from build123d import *

# Parameters (mm, degrees)
SKETCH_1_W          = 72
SKETCH_1_H          = 16
EXTRUDE_1_DEPTH     = 1.2
FILLET_1_R          = 3
CUT_EXTRUDE_1_REACH = 75.766
SKETCH_3_R          = 1.2


with BuildPart() as part:
    # 草图1 → 凸台-拉伸1 (new body)
    with BuildSketch(Plane.XY):
        with Locations((36, 8)):
            Rectangle(SKETCH_1_W, SKETCH_1_H)
    extrude(amount=EXTRUDE_1_DEPTH)

    # 圆角1
    fillet_1_edges = [part.edges().sort_by_distance(p)[0] for p in [
        (0, 16, 0.6),
        (72, 16, 0.6),
        (72, 0, 0.6),
        (0, 0, 0.6),
    ]]
    fillet(fillet_1_edges, radius=FILLET_1_R)

    # 草图3 → 切除-拉伸1 (cut, up to next)
    with BuildSketch(Plane(origin=(0, 0, 0), x_dir=(-1, 0, 0), z_dir=(0, 0, -1)), mode=Mode.PRIVATE) as cut_extrude_1_sk1:
        with Locations((-70.012877826, 14.013032766)):
            Circle(SKETCH_3_R)
    cut_extrude_1_tool1 = extrude(cut_extrude_1_sk1.sketch, amount=-CUT_EXTRUDE_1_REACH, mode=Mode.PRIVATE) & part.part
    # 草图3 → 切除-拉伸1 (cut, up to next)
    with BuildSketch(Plane(origin=(0, 0, 0), x_dir=(-1, 0, 0), z_dir=(0, 0, -1)), mode=Mode.PRIVATE) as cut_extrude_1_sk2:
        with Locations((-70.012694945, 2.012672085)):
            Circle(SKETCH_3_R)
    cut_extrude_1_tool2 = extrude(cut_extrude_1_sk2.sketch, amount=-CUT_EXTRUDE_1_REACH, mode=Mode.PRIVATE) & part.part
    # 草图3 → 切除-拉伸1 (cut, up to next)
    with BuildSketch(Plane(origin=(0, 0, 0), x_dir=(-1, 0, 0), z_dir=(0, 0, -1)), mode=Mode.PRIVATE) as cut_extrude_1_sk3:
        with Locations((-2.011949988, 14.012003328)):
            Circle(SKETCH_3_R)
    cut_extrude_1_tool3 = extrude(cut_extrude_1_sk3.sketch, amount=-CUT_EXTRUDE_1_REACH, mode=Mode.PRIVATE) & part.part
    # 草图3 → 切除-拉伸1 (cut, up to next)
    with BuildSketch(Plane(origin=(0, 0, 0), x_dir=(-1, 0, 0), z_dir=(0, 0, -1)), mode=Mode.PRIVATE) as cut_extrude_1_sk4:
        with Locations((-2.012501905, 2.013009906)):
            Circle(SKETCH_3_R)
    cut_extrude_1_tool4 = extrude(cut_extrude_1_sk4.sketch, amount=-CUT_EXTRUDE_1_REACH, mode=Mode.PRIVATE) & part.part
    add(cut_extrude_1_tool1.solids().sort_by_distance((70.012878, 14.013033, 0))[0], mode=Mode.SUBTRACT)
    add(cut_extrude_1_tool2.solids().sort_by_distance((70.012695, 2.012672, 0))[0], mode=Mode.SUBTRACT)
    add(cut_extrude_1_tool3.solids().sort_by_distance((2.01195, 14.012003, 0))[0], mode=Mode.SUBTRACT)
    add(cut_extrude_1_tool4.solids().sort_by_distance((2.012502, 2.01301, 0))[0], mode=Mode.SUBTRACT)


solid = part.part
Part model, mm, in its own coordinate system. Give positions to 0.01 mm unless a question says otherwise; leave off trailing zeros. Order: outer loops, then holes, each group sorted by start corner. A loop starts at its lowest first (then second) coordinate and runs counter-clockwise, first axis right, second up. Notation, with made-up numbers: (25.5, 11) - (84.5, 11) arc R10 cw to (84.5, 22) - close; hole circle Ø10 at (42.5, 55.25). An arc over 180 degrees is marked (long way). Use a Markdown table: item, result.
1) Flat gauge pin, fed straight in: P1, Ø1.9, axis at x = 2.01, y = 14.01, coming from the -Z side. Where does the tip first touch, or does it go through?
Checked values:
| item | result |
|---|---|
| P1 | through |
2) Saw through at A-A on z = 0.5. List the corners of the cut face in (x, y), plus the area to 3 significant figures.
Checked values:
| item | result |
|---|---|
| outline | (0, 3) arc R3 ccw to (3, 0) - (69, 0) arc R3 ccw to (72, 3) - (72, 13) arc R3 ccw to (69, 16) - (3, 16) arc R3 ccw to (0, 13) - close; hole circle Ø2.4 at (2.01, 2.01); hole circle Ø2.4 at (2.01, 14.01); hole circle Ø2.4 at (70.01, 2.01); hole circle Ø2.4 at (70.01, 14.01) |
| area | 1,130 mm² |
3) Probe L1, parallel to X at y = 3, z = 0.1; L2, parallel to X at y = 15, z = 0.1. List the from-to ranges inside material, lowest first. Write a range as from..to.
Checked values:
| item | result |
|---|---|
| L1 | 0..1.33, 2.7..69.33, 70.69..72 |
| L2 | 0.76..1.33, 2.69..69.33, 70.7..71.24 |
4) Two-plate mould, pull along X, no slides. Class faces 1 (the flat face through (36, 0, 1)), 2 (the cylindrical face through (2.17, 15.2, 0.59)), 3 (the flat face through (0, 8, 1)): +X half, -X half, draft (parallel to the pull), parting line (faces both ways), or undercut.
Checked values:
| item | result |
|---|---|
| face 1 | draft |
| face 2 | undercut |
| face 3 | -X half |
